Could you check a few things on this model? Use its own coordinates, in mm. Give positions to 0.01 mm unless a question says otherwise; leave off trailing zeros. Order: outer loops, then holes, each group sorted by start corner. A loop starts at its lowest first (then second) coordinate and runs counter-clockwise, first axis right, second up. Notation, with made-up numbers: (29.25, 81.5) - (39.25, 81.5) arc R9 ccw to (39.25, 95.5) - close; hole circle Ø4 at (76, -1). An arc over 180 degrees is marked (long way). One line per question, with ' | ' between items. Start each with the question number.
1. Imagine slicing it at B-B (x = 0). Please give me the cut outline in (y, z).
2. For P1, Ø4, axis at x = 7, z = 5, coming from the -Y side, with a flat end and sliding along its axis, tell me the tip position at first contact or that it passes through.
3. Imagine slicing it at A-A (y = 3.5). Please give me the cut outline in (x, z).
4. If we mould it in two halves opening along X, with no side actions, what happens to faces 1 (the flat face through (-11.05, 6.26, -6.26)), 2 (the flat face through (-3, 0, 6)), 3 (the flat face through (10.947, 6.261, -6.439)), 4 (the cylindrical face through (1.38, 6.26, 6.2))? For each: released by +X, released by -X, zero draft, split by the parting line, or undercut.
5. Imagine slicing it at D-D (z = -10.75). Please give me the cut outline in (x, y), and give its area (3 significant figures).
6. I need wall thicknesses on probe 1 along Z at (x, y) = (0, 6); probe 2 along X at (y, z) = (6.25, 3.5); probe 3 along Z at (x, y) = (-5.25, 10.75). Which ranges of each line are inside material? Lowest first, please. Write a range as from..to.
7. Imagine slicing it at C-C (z = 1.75). Please give me the cut outline in (x, y), and give its area (3 significant figures).
Autodesk Inventor part; units mm, degrees
ref_plane "YZ Plane" through (0, 0, 0) normal (1, 0, 0) x (0, 1, 0)
ref_plane "XZ Plane" through (0, 0, 0) normal (0, 1, 0) x (-1, 0, 0)
ref_plane "XY Plane" through (0, 0, 0) normal (0, 0, 1) x (1, 0, 0)
sketch "Sketch1" plane through (0, 0, 0) normal (0, 1, 0) x (-1, 0, 0)
  line L0 (-14.6647, 0) -> (-7.3323, 12.7)
  line L1 (-7.3323, 12.7) -> (7.3323, 12.7)
  line L2 (7.3323, 12.7) -> (14.6647, 0)
  line L3 (14.6647, 0) -> (7.3323, -12.7)
  line L4 (7.3323, -12.7) -> (-7.3323, -12.7)
  line L5 (-7.3323, -12.7) -> (-14.6647, 0)
  circle A0 centre (0, 0) radius 6.35
  dimension "d0" = 25.4
  dimension "d1" = 12.7
extrude "Extrusion1" add sketch "Sketch1" along normal blind 12.7
sketch "Sketch2" plane through (-7.3323, 0, 12.7) normal (0, 0, 1) x (1, 0, 0)
  point P0 (7.3323, 0)
properties part number "printCalibration"
Results found:
1) outline: (0, -12.7) - (12.7, -12.7) - (12.7, -6.35) - (0, -6.35) - close; (0, 6.35) - (12.7, 6.35) - (12.7, 12.7) - (0, 12.7) - close
2) P1: stops at y = 0
3) outline: (-14.66, 0) - (-7.33, -12.7) - (7.33, -12.7) - (14.66, 0) - (7.33, 12.7) - (-7.33, 12.7) - close; hole circle Ø12.7 at (0, 0)
4) face 1: released by -X | face 2: zero draft | face 3: released by +X | face 4: undercut
5) outline: (-8.46, 0) - (8.46, 0) - (8.46, 12.7) - (-8.46, 12.7) - close | area: 215 mm2
6) probe 1: z = -12.7..-6.35, 6.35..12.7 | probe 2: x = -12.64..-5.3, 5.3..12.64 | probe 3: z = -12.7..-3.57, 3.57..12.7
7) outline: (-13.65, 0) - (-6.1, 0) - (-6.1, 12.7) - (-13.65, 12.7) - close; (6.1, 0) - (13.65, 0) - (13.65, 12.7) - (6.1, 12.7) - close | area: 192 mm2
